Geometry: see drawing. Coordinates: mm, zero at the bounding-box minimum. Round coordinates to 2 decimals unless told otherwise and drop trailing zeros. Order: outer loops, then holes, each group sorted by start corner. A loop starts at its lowest first (then second) coordinate and runs counter-clockwise, first axis right, second up. Notation, with made-up numbers: (-32, 6.5) -> (-3, 6.5) arc R26 cw to (-3, 28.5) -> close; hole circle Ø8 at (0.5, 66.5). An arc over 180 degrees is marked (long way). One line per item, written item: value. Start each with the question number.
1) Section A-A (z = 9.25). Return the cut outline in (x, y), and give its area (3 significant figures).
2) Section B-B (x = 5.75). Return the cut outline in (y, z).
3) Ray query, L1, parallel to Z at x = 4, y = 32.5; L2, parallel to Y at x = 22.25, z = 15.25; L3, parallel to X at y = 4.5, z = 12. Return the intervals inside material, ascending.
4) Section C-C (y = 8). Return the cut outline in (x, z).
5) Section D-D (x = 11.5). Return the cut outline in (y, z).
6) Mould query, pull axis Y, two halves, no side actions, for the marked faces 1, 2, 3 and 4. Classes: pulls with the +Y half, pulls with the -Y half, needs draft (parallel to the pull), parting line crosses it, or undercut.
7) Pin query (flat end, axial travel): P1, Ø3, axis at y = 29.5, z = 17.5, coming from the -X side; P2, Ø1.6, axis at x = 9, z = 4, coming from the -Y side; P3, Ø3, axis at x = 12, z = 7, coming from the +Y side; P4, Ø1.6, axis at x = 14, z = 17, coming from the -Y side. Return the tip coordinate at first contact, or that it passes through.
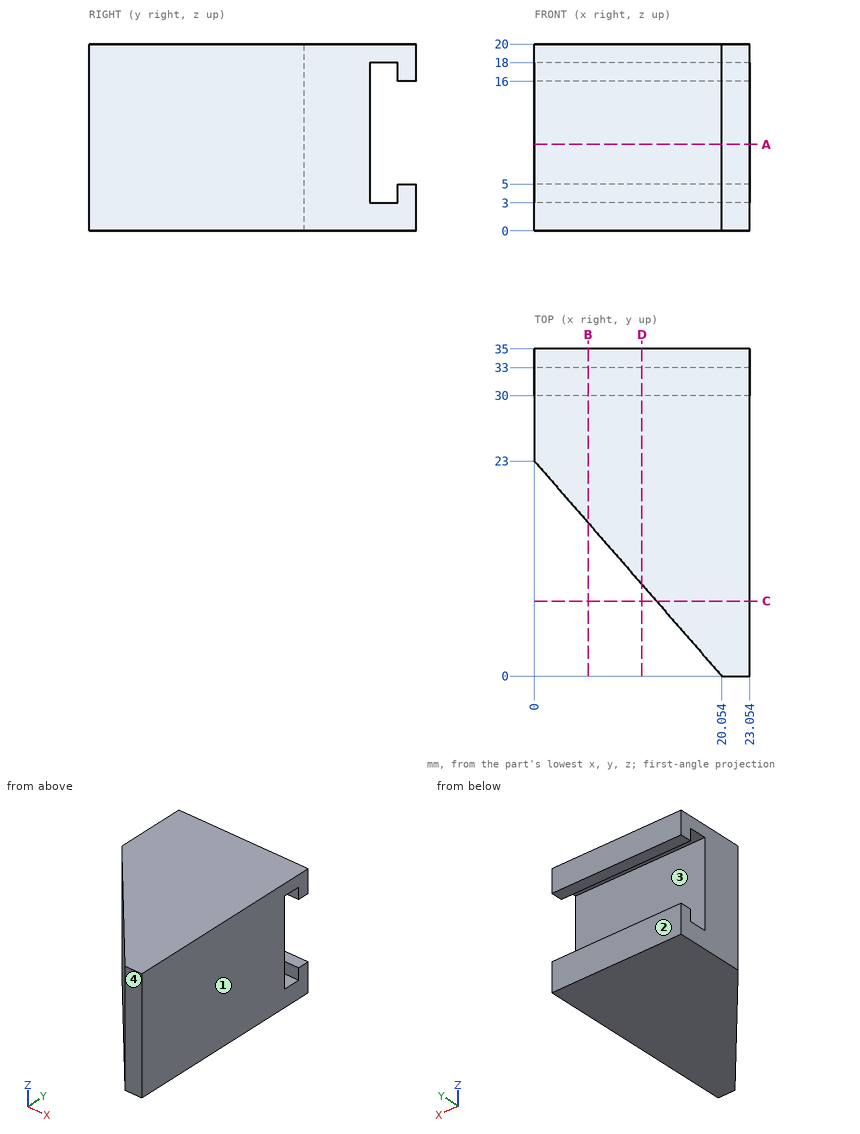
Findings:
1. outline: (0, 23) -> (20.05, 0) -> (23.05, 0) -> (23.05, 30) -> (0, 30) -> close
1. area: 461 mm2
2. outline: (16.41, 0) -> (35, 0) -> (35, 5) -> (33, 5) -> (33, 3) -> (30, 3) -> (30, 18) -> (33, 18) -> (33, 16) -> (35, 16) -> (35, 20) -> (16.41, 20) -> close
3. L1: 0 to 3, 18 to 20
3. L2: 0 to 30
3. L3: 16.13 to 23.05
4. outline: (13.08, 0) -> (23.05, 0) -> (23.05, 20) -> (13.08, 20) -> close
5. outline: (9.81, 0) -> (35, 0) -> (35, 5) -> (33, 5) -> (33, 3) -> (30, 3) -> (30, 18) -> (33, 18) -> (33, 16) -> (35, 16) -> (35, 20) -> (9.81, 20) -> close
6. face 1: needs draft
6. face 2: pulls with the +Y half
6. face 3: undercut
6. face 4: pulls with the -Y half
7. P1: x = 0
7. P2: y = 11.76
7. P3: y = 30
7. P4: y = 6.03
